from build123d import *

# Parameters (mm, degrees)
F0_R     = 17
F0_R_2   = 11.25
F1_DEPTH = 40


with BuildPart() as f1:
    # F0 (on Top) → F1 (new body)
    with BuildSketch(Plane.XY):
        Circle(F0_R)
        with BuildLine():
            ThreePointArc((-9, -6.5), (-9.146447, -6.853553), (-9.5, -7))
            Line((-9.5, -7), (-14.5, -7))
            ThreePointArc((-14.5, -7), (-14.853553, -6.853553), (-15, -6.5))
            Line((-15, -6.5), (-15, 6.5))
            ThreePointArc((-15, 6.5), (-14.853553, 6.853553), (-14.5, 7))
            Line((-14.5, 7), (-9.5, 7))
            ThreePointArc((-9.5, 7), (-9.146447, 6.853553), (-9, 6.5))
            Line((-9, 6.5), (-9, -6.5))
        make_face(mode=Mode.SUBTRACT)
        with Locations((3.75, 0)):
            Circle(F0_R_2, mode=Mode.SUBTRACT)
    extrude(amount=F1_DEPTH)


solid = f1.part
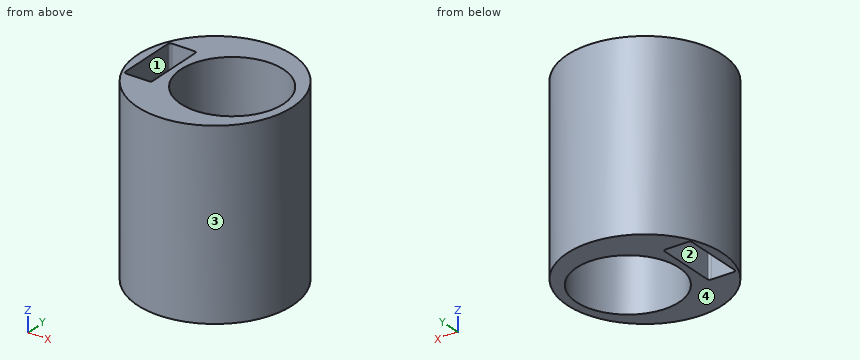
Can you work these out from the model? Positions are in its coordinate system, mm. Face numbers are marked on the shaded views. Coordinates: 2 decimals unless noted, no trailing zeros. Write each loop counter-clockwise with the first axis right and the second up, starting at its lowest first coordinate (ties: lowest second). Pieces come first, ordered by that corner, then holes. Notation, with made-up numbers: (-19, -17.5) - (29, -17.5) arc R21 ccw to (29, 16.5) - close; hole circle Ø11 at (-22.75, -14). An arc over 180 degrees is marked (long way). Return JSON: item names as keys, results as strings. Group by question number.
Item 1: We'd pull the mould along X, two halves only. Please class the marked faces 1, 2, 3 and 4: pulls with the +X half, pulls with the -X half, needs draft (parallel to the pull), parting line crosses it, or undercut.
Item 2: If we section it at A-A (z = 4): Write out the boundary of the cut face in (x, y), then the cut area to 3 significant figures.
Item 3: If we section it at C-C (x = 1): Write out the boundary of the cut face in (y, z).
Item 4: Please list where these lines run through material, in increasing order: probe 1 along X at (y, z) = (-3, 13); probe 2 along X at (y, z) = (5, 13); probe 3 along Y at (x, z) = (3.75, 13).
Item 5: I'm going to push flat-ended pins straight in: pin 1 Ø4 at (x, z) = (-11.5, 21.5) entering from -Y; pin 2 Ø3 at (y, z) = (9, 25.5) entering from -X; pin 3 Ø1 at (y, z) = (11.5, 17.5) entering from -X; pin 4 Ø10 at (x, y) = (2, -3) entering from +Z. Where does each tip first touch, or does it pass through?
Item 6: If we section it at B-B (y = 0): Write out the boundary of the cut face in (x, z), then the cut area to 3 significant figures.
Item 7: If we section it at D-D (y = -8): Write out the boundary of the cut face in (x, z).
Return value:
{
 "1": {"face 1": "undercut", "face 2": "undercut", "face 3": "parting line crosses it", "face 4": "needs draft"},
 "2": {"outline": "circle Ø34 at (0, 0); hole (-15, -6.5) arc R0.5 ccw to (-14.5, -7) - (-9.5, -7) arc R0.5 ccw to (-9, -6.5) - (-9, 6.5) arc R0.5 ccw to (-9.5, 7) - (-14.5, 7) arc R0.5 ccw to (-15, 6.5) - close; hole circle Ø22.5 at (3.75, 0)", "area": "427 mm^2"},
 "3": {"outline": "(-16.97, 0) - (-10.91, 0) - (-10.91, 40) - (-16.97, 40) - close; (10.91, 0) - (16.97, 0) - (16.97, 40) - (10.91, 40) - close"},
 "4": {"probe 1": "x = -16.73 to -15, -9 to -7.09, 14.59 to 16.73", "probe 2": "x = -16.25 to -15, -9 to -6.33, 13.83 to 16.25", "probe 3": "y = -16.58 to -11.25, 11.25 to 16.58"},
 "5": {"pin 1": "stops at y = -14.1", "pin 2": "stops at x = -15.26", "pin 3": "stops at x = -12.96", "pin 4": "passes through"},
 "6": {"outline": "(-17, 0) - (-15, 0) - (-15, 40) - (-17, 40) - close; (-9, 0) - (-7.5, 0) - (-7.5, 40) - (-9, 40) - close; (15, 0) - (17, 0) - (17, 40) - (15, 40) - close", "area": "220 mm^2"},
 "7": {"outline": "(-15, 0) - (-4.16, 0) - (-4.16, 40) - (-15, 40) - close; (11.66, 0) - (15, 0) - (15, 40) - (11.66, 40) - close"}
}
